Read the model definition and answer for the solid it produces. Units are mm, in the model's axes. Face numbers are marked on the shaded views. A direction names the side the tool comes from. Give positions to 0.01 mm unless a question says otherwise; leave off trailing zeros. Order: outer loops, then holes, each group sorted by start corner. A loop starts at its lowest first (then second) coordinate and runs counter-clockwise, first axis right, second up. Notation, with made-up numbers: (7.5, -33) -> (42.5, -33) arc R27 cw to (42.5, -5) -> close; hole circle Ø5 at (2.25, 28). An arc over 180 degrees is marked (long way). Use one line per item in the form item = value.
```python
from build123d import *

# Parameters (mm, degrees)
SKETCH1_W           = 80
SKETCH1_H           = 20
BOSS_EXTRUDE1_DEPTH = 5
SKETCH2_R           = 2.75
CUT_EXTRUDE1_DEPTH  = 5
SKETCH3_W           = 61
SKETCH3_H           = 13
SKETCH3_R           = 2.25
BOSS_EXTRUDE2_DEPTH = 3
SKETCH4_W           = 3
SKETCH4_H           = 13
BOSS_EXTRUDE3_DEPTH = 17
SKETCH5_R           = 7.771284408
CUT_EXTRUDE2_DEPTH  = 17


with BuildPart() as part:
    # Sketch1 → Boss-Extrude1 (new body)
    with BuildSketch(Plane(origin=(0, 0, 0), x_dir=(1, 0, 0), z_dir=(0, 1, 0))):
        Rectangle(SKETCH1_W, SKETCH1_H)
    extrude(amount=BOSS_EXTRUDE1_DEPTH)

    # Sketch2 → Cut-Extrude1 (cut)
    with BuildSketch(Plane(origin=(0, 5, 0), x_dir=(1, 0, 0), z_dir=(0, 1, 0))):
        with Locations((-34, 0)):
            Circle(SKETCH2_R)
        with Locations((34, 0)):
            Circle(SKETCH2_R)
    extrude(amount=-CUT_EXTRUDE1_DEPTH, mode=Mode.SUBTRACT)

    # Sketch3 → Boss-Extrude2 (add)
    with BuildSketch(Plane.XY.offset(10)):
        with Locations((0, 11.5)):
            Rectangle(SKETCH3_W, SKETCH3_H)
        with Locations((-21, 11.5)):
            Circle(SKETCH3_R, mode=Mode.SUBTRACT)
        with Locations((21, 11.5)):
            Circle(SKETCH3_R, mode=Mode.SUBTRACT)
    extrude(amount=-BOSS_EXTRUDE2_DEPTH)

    # Sketch4 → Boss-Extrude3 (add)
    with BuildSketch(Plane(origin=(0, 0, 7), x_dir=(-1, 0, 0), z_dir=(0, 0, -1))):
        with Locations((-29, 11.5)):
            Rectangle(SKETCH4_W, SKETCH4_H)
        with Locations((29, 11.5)):
            Rectangle(SKETCH4_W, SKETCH4_H)
    extrude(amount=BOSS_EXTRUDE3_DEPTH)

    # Sketch5 → Cut-Extrude2 (cut)
    with BuildSketch(Plane(origin=(0, 5, 0), x_dir=(1, 0, 0), z_dir=(0, 1, 0))):
        with Locations((0, 10)):
            Circle(SKETCH5_R)
    extrude(amount=-CUT_EXTRUDE2_DEPTH, mode=Mode.SUBTRACT)


solid = part.part
```
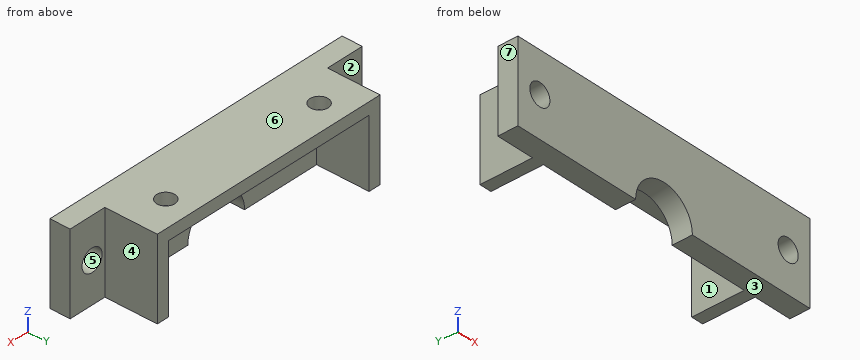
Item 1: The part is cut by section B-B on x = -34. Give the vertices of the cut face in (y, z), and give its area (3 significant figures).
Checks:
outline = (0, -10) -> (5, -10) -> (5, -2.75) -> (0, -2.75) -> close; (0, 2.75) -> (5, 2.75) -> (5, 10) -> (0, 10) -> close
area = 72.5 mm²
Item 2: Which of the six approach directions +Z, -Z, +X, -X, +Y, -Y give full straight-line access (tool end or side, diameter ignored) to the marked faces 1, 2, 3 and 4?
Checks:
face_1 = -Z, +Y
face_2 = +Z, -Z, -X, +Y
face_3 = -Z, +X, -X, +Y, -Y
face_4 = +Z, -Z, +X, +Y
Item 3: Determine the mould class of the marked faces 5, 6 and 7 for opening direction Z: +Z half, -Z half, draft (parallel to the pull), parting line (faces both ways), or undercut.
Checks:
face_5 = undercut
face_6 = +Z half
face_7 = draft
Item 4: Straight lines are drawn through the part: L1, parallel to X at y = 1.75, z = 0; L2, parallel to X at y = 11.25, z = 0; L3, parallel to Z at x = 34, y = 4.05. For each, find the intervals that lie inside material, in ascending order. Write a range as from..to.
Checks:
L1 = -40..-36.75, -31.25..31.25, 36.75..40
L2 = -30.5..-27.5, 27.5..30.5
L3 = -10..-2.75, 2.75..10
Item 5: The part is cut by section A-A on z = 0. Give the vertices of the cut face in (x, y), and give its area (3 significant figures).
Checks:
outline = (-40, 0) -> (-36.75, 0) -> (-36.75, 5) -> (-40, 5) -> close; (-31.25, 0) -> (31.25, 0) -> (31.25, 5) -> (30.5, 5) -> (30.5, 18) -> (27.5, 18) -> (27.5, 5) -> (-27.5, 5) -> (-27.5, 18) -> (-30.5, 18) -> (-30.5, 5) -> (-31.25, 5) -> close; (36.75, 0) -> (40, 0) -> (40, 5) -> (36.75, 5) -> close
area = 423 mm²
Item 6: The part is cut by section D-D on y = 7.25. Give the vertices of the cut face in (x, z).
Checks:
outline = (-30.5, -10) -> (-27.5, -10) -> (-27.5, 7) -> (27.5, 7) -> (27.5, -10) -> (30.5, -10) -> (30.5, 10) -> (-30.5, 10) -> close
Item 7: The part is cut by section C-C on z = 5.25. Give the vertices of the cut face in (x, y), and give its area (3 significant figures).
Checks:
outline = (-40, 0) -> (40, 0) -> (40, 5) -> (30.5, 5) -> (30.5, 18) -> (27.5, 18) -> (27.5, 5) -> (-27.5, 5) -> (-27.5, 18) -> (-30.5, 18) -> (-30.5, 5) -> (-40, 5) -> close
area = 478 mm²
Item 8: Given pin 1 Ø5 at (x, z) = (-34, 0) entering from +Y; pin 2 Ø8 at (x, z) = (-6.5, -7.5) entering from -Y; pin 3 Ø6 at (y, z) = (10, 7.5) entering from -X; pin 4 Ø10.5 at (y, z) = (13, -1.5) entering from +X, each flat-ended and moving along its own axis, determine where each tip first touches the part or whether it passes through.
Checks:
pin_1 = through
pin_2 = 0
pin_3 = -30.5
pin_4 = 30.5
